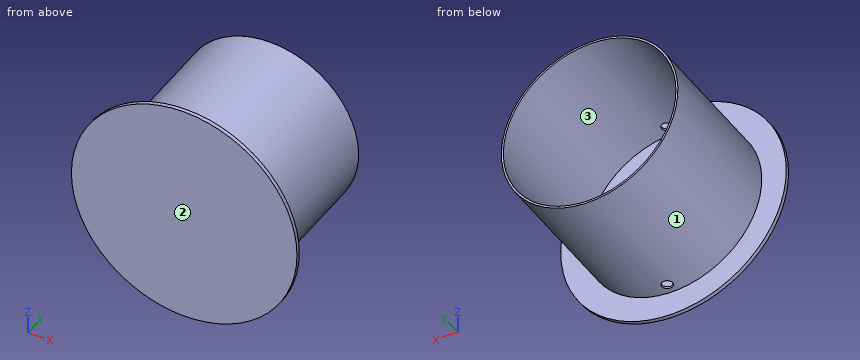
from build123d import *

# Parameters (mm, degrees)
BASE_FLANGE_SKETCH_R       = 230
BASE_FLANGE_DEPTH          = 8
TANK_WALL_SKETCH_R         = 180
TANK_WALL_SKETCH_R_2       = 176
TANK_WALL_DEPTH            = 300
TAP_DRAIN_PORTS_DEPTH      = 443.492937797
TAP_DRAIN_PORTS_DEPTH_BACK = 443.492937797
PORT_HOLES_SKETCH_R        = 11


with BuildPart() as part:
    # Base Flange Sketch → Base Flange (new body)
    with BuildSketch(Plane(origin=(0, 0, 0), x_dir=(1, 0, 0), z_dir=(0, 1, 0))):
        with Locations(Location((0, 0, 0), (0, 0, 270))):
            Circle(BASE_FLANGE_SKETCH_R)
    extrude(amount=BASE_FLANGE_DEPTH)

    # Tank Wall Sketch → Tank Wall (add)
    with BuildSketch(Plane(origin=(0, 0, 0), x_dir=(1, 0, 0), z_dir=(0, 1, 0))):
        with Locations(Location((0, 0, 0), (0, 0, 270))):
            Circle(TANK_WALL_SKETCH_R)
        with Locations(Location((0, 0, 0), (0, 0, 270))):
            Circle(TANK_WALL_SKETCH_R_2, mode=Mode.SUBTRACT)
    extrude(amount=TANK_WALL_DEPTH)

    # Port Holes Sketch → Tap + Drain Ports (cut, two sides: drawn at the far end of the back side and taken through both)
    with BuildSketch(Plane.XY.offset(-TAP_DRAIN_PORTS_DEPTH_BACK)):
        with Locations((0, 30)):
            Circle(PORT_HOLES_SKETCH_R)
    extrude(amount=TAP_DRAIN_PORTS_DEPTH + TAP_DRAIN_PORTS_DEPTH_BACK, mode=Mode.SUBTRACT)


solid = part.part
Could you check a few things on this model? Use its own coordinates, in mm. Face numbers are marked on the shaded views. Give positions to 0.01 mm unless a question says otherwise; leave off trailing zeros. Order: outer loops, then holes, each group sorted by start corner. A loop starts at its lowest first (then second) coordinate and runs counter-clockwise, first axis right, second up. Notation, with made-up numbers: M -13.5,29 L 12.5,29 A16 ccw 12.5,48 Z; hole C -5.5,30.5 d1. An arc over 180 degrees is marked long. One line per question, with ' | ' between items.
1. I'm going to push flat-ended pins straight in: pin 1 (4 mm diameter, centred on x = -29.5, z = 153.5, fed in from +Y); pin 2 (12 mm diameter, centred on x = 80.5, y = 81, fed in from +Z); pin 3 (13 mm diameter, centred on x = 0, y = 30, fed in from +Z) (3 decimals); pin 4 (8 mm diameter, centred on x = 76.5, y = 151, fed in from +Z). Where does each tip first touch, or does it pass through?
Results:
pin 1: y = 8 | pin 2: z = 163.86 | pin 3: through | pin 4: z = 164.75
2. I want a section at C-C (z = 0). List the corners of the cut face in (x, y) for me.
Results:
outline: M -230,0 L 230,0 L 230,8 L 180,8 L 180,300 L 176,300 L 176,8 L -176,8 L -176,300 L -180,300 L -180,8 L -230,8 Z
3. I want a section at A-A (x = 0). List the corners of the cut face in (y, z) for me, and give its area (3 significant figures).
Results:
outline: M 0,-230 L 8,-230 L 8,-180 L 19,-180 L 19,-176 L 8,-176 L 8,176 L 19,176 L 19,180 L 8,180 L 8,230 L 0,230 Z; M 41,-180 L 300,-180 L 300,-176 L 41,-176 Z; M 41,176 L 300,176 L 300,180 L 41,180 Z | area: 5,840 mm²
4. I want a section at D-D (y = 89). List the corners of the cut face in (x, z) for me.
Results:
outline: C 0,0 d360; hole C 0,0 d352
5. If I drill on line 1 (Z direction, x = 0, y = 225); line 2 (Y direction, x = -208, z = 76.5), over which ranges is the centre line in solid material (lowest first)?
Results:
line 1: -180 to -176, 176 to 180 | line 2: 0 to 8
6. We'd pull the mould along X, two halves only. Please class the marked faces 1, 2 and 3: +X half, -X half, draft (parallel to the pull), parting line (faces both ways), or undercut.
Results:
face 1: parting line | face 2: draft | face 3: undercut
